Design review of the part built by this model. Coordinates are the model's own, in mm. A direction names the side the tool comes from. Give positions to 0.01 mm unless a question says otherwise; leave off trailing zeros. Loops run counter-clockwise (first coordinate to the right, second up) from the corner with the lowest first, then second, coordinate; pieces in that order, holes last. Notation, with made-up numbers: (73.25, 87) -> (102.25, 87) arc R24 cw to (102.25, 118) -> close; hole circle Ø2 at (19.25, 16). An arc over 180 degrees is marked (long way). Use CSV: the item, a comma, the result in double quotes. Start each with the question number.
Item 1: Wall thickness on line 1 along Z through (x, y) = (1, 74.5); line 2 along Y through (x, z) = (1.75, -0.75) (3 decimals); line 3 along Y through (x, z) = (0.5, -3): over which ranges is each line inside the solid? List them lowest first. Write a range as from..to.
Item 2: For faces 5 (the face through (3.3, 77.5, 0.9)), 6 (the face through (-6.49, 73.34, -6.02)), 7 (the face through (-4, 75, 0)), list the 3-axis set-ups (+Z, -Z, +X, -X, +Y, -Y) from which the entire face can be reached by the end or side of a thin tool; tool diameter is ignored.
Item 3: We need section A-A (x = -1.5). State the section outline as (y, z) points.
Item 4: We need section B-B (y = 81.5). State the section outline as (x, z) points.
Item 5: Clearance check with flat-ended pins moving along their axes: pin 1 (4.5 mm diameter, centred on x = -0.5, y = 76.5, fed in from -Z); pin 2 (1 mm diameter, centred on x = -6, z = -0.5, fed in from -Y); pin 3 (2 mm diameter, centred on x = 0.5, y = 73.5, fed in from +Z); pin 4 (4 mm diameter, centred on y = 82, z = -2, fed in from -X). State where each tip first meets the part, or that it passes through.
Item 6: The part is to be moulded in two halves that separate along X. For faces 1 (the face through (-0.159, 82.215, -1.306)), 2 (the face through (3.418, 73.264, -2.282)), 3 (the face through (-2, 78, -4.5)), 4 (the face through (-6.74, 80.86, -2.28)), say which applies: +X half, -X half, draft (parallel to the pull), parting line (faces both ways), or undercut.
Item 7: We need section C-C (z = -1). State the section outline as (x, y) points.
Item 8: We need section D-D (y = 71). State the section outline as (x, z) points, plus the area to 3 significant figures.
from build123d import *
from build123d.topology import SkipClean

# Parameters (mm, degrees)
SKETCH3_R           = 2.75
SKETCH3_R_2         = 2.1
BOSS_EXTRUDE2_DEPTH = 11
BOSS_EXTRUDE4_START = 4.5
BOSS_EXTRUDE4_DEPTH = 4.5
BOSS_EXTRUDE3_START = 3
BOSS_EXTRUDE3_DEPTH = 3
SKETCH14_W          = 47.285712055
SKETCH14_H          = 12.595473758
CUT_EXTRUDE1_DEPTH  = 92.326119258
BOSS_EXTRUDE5_DEPTH = 1.8
SKETCH15_R          = 2.1
CUT_EXTRUDE2_DEPTH  = 88.749019959


with BuildPart() as part:
    # Sketch3 → Boss-Extrude2 (new body)
    with BuildSketch(Plane.XY):
        with BuildLine():
            Line((11.81639044, 60.252883085), (11.728372068, 60.311638564))
            ThreePointArc((11.728372068, 60.311638564), (8.917204522, 62.7925154), (6.866230988, 65.931132995))
            ThreePointArc((6.866230988, 65.931132995), (6.025591445, 67.274340702), (4.901176311, 68.390840765))
            ThreePointArc((4.901176311, 68.390840765), (3.375934297, 70.989881123), (4.020351516, 73.93370524))
            Line((4.020351516, 73.93370524), (5.678869184, 76.41823992))
            ThreePointArc((5.678869184, 76.41823992), (3.137547336, 86.100651278), (-6.171856019, 82.420649156))
            Line((-6.171856019, 82.420649156), (-7.290261888, 79.347854286))
            ThreePointArc((-7.290261888, 79.347854286), (-8.557893098, 69.185727028), (-5.279809822, 59.483671095))
            ThreePointArc((-5.279809822, 59.483671095), (-2.848156457, 57.139360441), (0.414833066, 56.266646336))
            ThreePointArc((0.414833066, 56.266646336), (3.287818882, 55.822166382), (5.91364728, 54.574514525))
            Line((5.91364728, 54.574514525), (7.374782695, 53.599153256))
            ThreePointArc((7.374782695, 53.599153256), (10.815902262, 50.678650143), (13.499590609, 47.049812979))
            ThreePointArc((13.499590609, 47.049812979), (24.965953819, 46.665736496), (20.21385057, 57.108078892))
            ThreePointArc((20.21385057, 57.108078892), (15.833272198, 58.194897845), (11.81639044, 60.252883085))
        make_face()
        with Locations((19.351869275, 50.413343031)):
            Circle(SKETCH3_R, mode=Mode.SUBTRACT)
        with Locations((0.471910886, 63.016405008)):
            Circle(SKETCH3_R, mode=Mode.SUBTRACT)
        with Locations((0.114687614, 80.132534397)):
            Circle(SKETCH3_R_2, mode=Mode.SUBTRACT)
    extrude(amount=BOSS_EXTRUDE2_DEPTH)

    # Sketch13 → Boss-Extrude4 (add)
    with SkipClean():  # the faces are left unmerged after this step: merging them gives an invalid solid
        with BuildSketch(Plane(origin=(0, 0, 0), x_dir=(-1, 0, 0), z_dir=(0, 0, -1)).offset(BOSS_EXTRUDE4_START)):
            with BuildLine():
                Line((-5.678869184, 76.41823992), (-4.020351516, 73.93370524))
                ThreePointArc((-4.020351516, 73.93370524), (-3.407782277, 73.255690271), (-2.625844204, 72.782913134))
                Line((-2.625844204, 72.782913134), (8.427696777, 68.139691908))
                ThreePointArc((8.427696777, 68.139691908), (8.557268078, 73.814637343), (7.290261888, 79.347854286))
                Line((7.290261888, 79.347854286), (6.171856019, 82.420649156))
                ThreePointArc((6.171856019, 82.420649156), (-3.137547336, 86.100651278), (-5.678869184, 76.41823992))
            make_face()
        extrude(amount=-BOSS_EXTRUDE4_DEPTH)

    # Sketch12 → Boss-Extrude3 (add)
    with SkipClean():  # the faces are left unmerged after this step: merging them gives an invalid solid
        with BuildSketch(Plane(origin=(0, 0, -4.5), x_dir=(-1, 0, 0), z_dir=(0, 0, -1)).offset(BOSS_EXTRUDE3_START)):
            with BuildLine():
                Line((8.013597957, 76.965805827), (4.924247842, 69.611373108))
                Line((4.924247842, 69.611373108), (8.427696777, 68.139691908))
                ThreePointArc((8.427696777, 68.139691908), (8.649339764, 72.572862025), (8.013597957, 76.965805827))
            make_face()
        extrude(amount=-BOSS_EXTRUDE3_DEPTH)

    # Sketch14 → Cut-Extrude1 (cut, through all)
    with BuildSketch(Plane(origin=(0, 0, 0), x_dir=(1, 0, 0), z_dir=(0, 1, 0))):
        with Locations((8.412006537, -6.297736879)):
            Rectangle(SKETCH14_W, SKETCH14_H)
    extrude(amount=CUT_EXTRUDE1_DEPTH, mode=Mode.SUBTRACT)

    # Sketch16 → Boss-Extrude5 (add)
    with BuildSketch(Plane.XY):
        with BuildLine():
            Line((3.739918762, 78.44206135), (2.852420412, 76.538814997))
            ThreePointArc((2.852420412, 76.538814997), (-2.463283783, 74.604056896), (-4.398041884, 79.919761091))
            Line((-4.398041884, 79.919761091), (-3.510543534, 81.823007444))
            ThreePointArc((-3.510543534, 81.823007444), (1.805160661, 83.757765545), (3.739918762, 78.44206135))
        make_face()
    extrude(amount=BOSS_EXTRUDE5_DEPTH)

    # Sketch15 → Cut-Extrude2 (cut, through all)
    with BuildSketch(Plane.XY.offset(1.8)):
        with Locations((0.114687614, 80.132534397)):
            Circle(SKETCH15_R)
    extrude(amount=-CUT_EXTRUDE2_DEPTH, mode=Mode.SUBTRACT)


solid = part.part
Results found:
1,line 1,"-4.5..0"
1,line 2,"72.415..78.815, 81.45..86.62"
1,line 3,"71.89..78.07, 82.2..86.81"
2,face 5,"+Z, +X, -Y"
2,face 6,"-Z, +X, +Y"
2,face 7,"+Z"
3,outline,"(71.05, -4.5) -> (78.79, -4.5) -> (78.79, 1.8) -> (74.3, 1.8) -> (74.3, 0) -> (71.05, 0) -> close; (81.48, -4.5) -> (86.62, -4.5) -> (86.62, 0) -> (83.79, 0) -> (83.79, 1.8) -> (81.48, 1.8) -> close"
4,outline,"(-6.51, -4.5) -> (-1.48, -4.5) -> (-1.48, 1.8) -> (-3.66, 1.8) -> (-3.66, 0) -> (-6.51, 0) -> close; (1.71, -4.5) -> (6.66, -4.5) -> (6.66, 0) -> (3.87, 0) -> (3.87, 1.8) -> (1.71, 1.8) -> close"
5,pin 1,"z = -4.5"
5,pin 2,"y = 68.95"
5,pin 3,"z = 1.8"
5,pin 4,"x = -7.05"
6,face 1,"undercut"
6,face 2,"+X half"
6,face 3,"draft"
6,face 4,"-X half"
7,outline,"(-8.43, 68.14) -> (2.63, 72.78) arc R3.14 ccw to (4.02, 73.93) -> (5.68, 76.42) arc R6.69 ccw (long way) to (-6.17, 82.42) -> (-7.29, 79.35) arc R22.95 ccw to start; hole circle Ø4.2 at (0.11, 80.13)"
8,outline,"(-8.67, -7.5) -> (-5.51, -7.5) -> (-5.51, -4.5) -> (-1.62, -4.5) -> (-1.62, 0) -> (-8.67, 0) -> close"
8,area,"41.2 mm²"
